```python
from build123d import *

# Parameters (mm, degrees)
SKETCH050_W      = 37
SKETCH050_H      = 132
PAD_DEPTH        = 6
PAD_DEPTH_BACK   = 4
SKETCH051_W      = 37
SKETCH051_H      = 119
POCKET006_DEPTH  = 4
HOLE_D           = 2.4
HOLE_DEPTH       = 25
HOLE_CBORE_D     = 3.5
HOLE_CBORE_DEPTH = 2.1
BINDER020_W      = 119
BINDER020_H      = 64
PAD012_DEPTH     = 6
SKETCH_R         = 1.75
POCKET_DEPTH     = 9
POCKET001_DEPTH  = 5
POCKET002_DEPTH  = 5
SKETCH046_R      = 1.75
POCKET003_DEPTH  = 4
POCKET004_DEPTH  = 5
SKETCH048_R      = 1.75
POCKET005_DEPTH  = 4


with BuildPart() as obj1:
    # Sketch050 (on Face1 of Binder) → Pad (new body, two sides)
    with BuildSketch(Plane.XY) as pad_sk:
        with Locations((-13.5, 0)):
            Rectangle(SKETCH050_W, SKETCH050_H)
    extrude(amount=PAD_DEPTH)
    extrude(pad_sk.sketch, amount=-PAD_DEPTH_BACK)

    # Sketch051 (on Face5 of Pad) → Pocket006 (cut)
    with BuildSketch(Plane(origin=(0, 0, -4), x_dir=(1, 0, 0), z_dir=(0, 0, -1))):
        with Locations((-13.5, 0)):
            Rectangle(SKETCH051_W, SKETCH051_H)
    extrude(amount=-POCKET006_DEPTH, mode=Mode.SUBTRACT)

    # Hole
    with Locations(Plane.XY.offset(6)):
        with Locations((-28.75, 62.75), (1.75, 62.75), (-28.75, -62.75), (1.75, -62.75)):
            CounterBoreHole(HOLE_D / 2, HOLE_CBORE_D / 2, HOLE_CBORE_DEPTH, depth=HOLE_DEPTH)


with BuildPart() as fusion:
    # Binder020 → Pad012 (new body)
    with BuildSketch(Plane(origin=(0, 0, 0), x_dir=(0, 1, 0), z_dir=(0, 0, 1))):
        Rectangle(BINDER020_W, BINDER020_H)
    extrude(amount=PAD012_DEPTH)

    # Sketch (on Face2 of Pad012) → Pocket (cut)
    with BuildSketch(Plane.YZ.offset(32)):
        with Locations((-34.5, 3)):
            Circle(SKETCH_R)
        with Locations((34.5, 3)):
            Circle(SKETCH_R)
    extrude(amount=-POCKET_DEPTH, mode=Mode.SUBTRACT)

    # Sketch044 (on Face3 of Pocket) → Pocket001 (cut)
    with BuildSketch(Plane.YZ.offset(32)):
        Polygon((-40.5, 0), (-38.316179, 6), (-30.683821, 6), (-28.5, 0), align=None)
        Polygon((30.683821, 6), (38.316179, 6), (40.5, 0), (28.5, 0), align=None)
    extrude(amount=-POCKET001_DEPTH, mode=Mode.SUBTRACT)

    # Sketch045 (on Face1 of Pocket001) → Pocket002 (cut)
    with BuildSketch(Plane.XZ.offset(59.5)):
        Polygon((10, 0), (12.183821, 6), (19.816179, 6), (22, 0), align=None)
    extrude(amount=-POCKET002_DEPTH, mode=Mode.SUBTRACT)

    # Sketch046 (on Face18 of Pocket002) → Pocket003 (cut)
    with BuildSketch(Plane.XZ.offset(54.5)):
        with Locations((16, 3)):
            Circle(SKETCH046_R)
    extrude(amount=-POCKET003_DEPTH, mode=Mode.SUBTRACT)

    # Sketch047 (on Face6 of Pocket003) → Pocket004 (cut)
    with BuildSketch(Plane(origin=(0, 59.5, 0), x_dir=(-1, 0, 0), z_dir=(0, 1, 0))):
        Polygon((-22, 0), (-19.816179, 6), (-12.183821, 6), (-10, 0), align=None)
    extrude(amount=-POCKET004_DEPTH, mode=Mode.SUBTRACT)

    # Sketch048 (on Face20 of Pocket004) → Pocket005 (cut)
    with BuildSketch(Plane(origin=(0, 54.5, 0), x_dir=(-1, 0, 0), z_dir=(0, 1, 0))):
        with Locations((-16, 3)):
            Circle(SKETCH048_R)
    extrude(amount=-POCKET005_DEPTH, mode=Mode.SUBTRACT)

    # Fusion: union obj1
    add(obj1.part)


solid = fusion.part
```
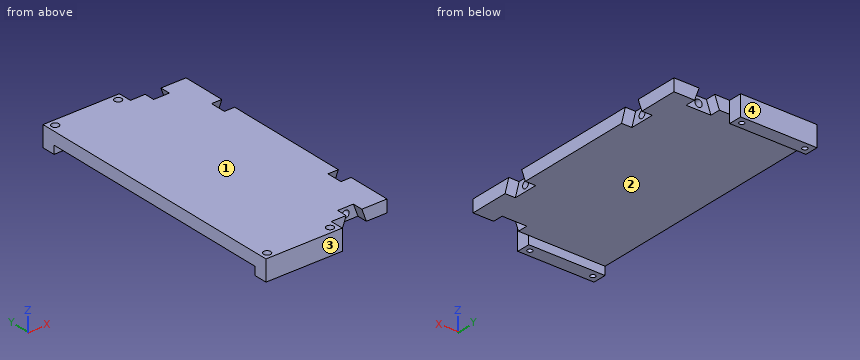
Part model, mm, in its own coordinate system. Face numbers are marked on the shaded views. Round coordinates to 2 decimals unless told otherwise and drop trailing zeros. Loops run counter-clockwise (first coordinate to the right, second up) from the corner with the lowest first, then second, coordinate; pieces in that order, holes last. Notation, with made-up numbers: (19, -18) -> (47, -18) arc R32 ccw to (47, 9) -> close; hole circle Ø2 at (11.25, 17). An arc over 180 degrees is marked (long way). Use one line per item in the form item = value. Start each with the question number.
Item 1: Band-saw the part on C-C (x = -28.75). List the corners of the cut face in (y, z), plus the area to 3 significant figures.
Item 2: Two-plate mould, pull along Y, no slides. Class the marked faces 1, 2, 3 and 4: released by +Y, released by -Y, zero draft, split by the parting line, or undercut.
Item 3: Band-saw the part on A-A (z = -1.5). List the corners of the cut face in (x, y).
Item 4: Drill centre lines: line 1 along Y through (x, z) = (1.75, 0.75); line 2 along Y through (x, z) = (1.75, 4.8); line 3 along Y through (x, z) = (-22.5, -3). Where is each one in solid material? Low to high.
Item 5: Band-saw the part on B-B (x = 16). List the corners of the cut face in (y, z), plus the area to 3 significant figures.
Item 6: Drop flat-ended pins along their axis: pin 1 Ø1.5 at (x, z) = (7, -1) entering from -Y; pin 2 Ø1.8 at (x, z) = (16, 3) entering from +Y; pin 3 Ø2 at (x, y) = (0.5, 16.5) entering from -Z; pin 4 Ø5 at (x, z) = (10, 2.5) entering from -Y. Give the stop position or say it passes through.
Item 7: Band-saw the part on D-D (y = -34.5). List the corners of the cut face in (x, z), plus the area to 3 significant figures.
Data:
q1.outline = (-66, -4) -> (-63.95, -4) -> (-63.95, 3.9) -> (-64.5, 3.9) -> (-64.5, 6) -> (-66, 6) -> close; (-61.55, -4) -> (-59.5, -4) -> (-59.5, 0) -> (59.5, 0) -> (59.5, -4) -> (61.55, -4) -> (61.55, 3.9) -> (61, 3.9) -> (61, 6) -> (-61, 6) -> (-61, 3.9) -> (-61.55, 3.9) -> close; (63.95, -4) -> (66, -4) -> (66, 6) -> (64.5, 6) -> (64.5, 3.9) -> (63.95, 3.9) -> close
q1.area = 791 mm^2
q2.face_1 = zero draft
q2.face_2 = undercut
q2.face_3 = released by -Y
q2.face_4 = released by +Y
q3.outline = (-32, -66) -> (5, -66) -> (5, -59.5) -> (-32, -59.5) -> close; (-32, 59.5) -> (5, 59.5) -> (5, 66) -> (-32, 66) -> close; hole circle Ø2.4 at (-28.75, -62.75); hole circle Ø2.4 at (-28.75, 62.75); hole circle Ø2.4 at (1.75, -62.75); hole circle Ø2.4 at (1.75, 62.75)
q4.line_1 = -66 to -63.95, -61.55 to 61.55, 63.95 to 66
q4.line_2 = -66 to -64.5, -61 to 61, 64.5 to 66
q4.line_3 = -66 to -59.5, 59.5 to 66
q5.outline = (-54.5, 0) -> (54.5, 0) -> (54.5, 1.25) -> (50.5, 1.25) -> (50.5, 4.75) -> (54.5, 4.75) -> (54.5, 6) -> (-54.5, 6) -> (-54.5, 4.75) -> (-50.5, 4.75) -> (-50.5, 1.25) -> (-54.5, 1.25) -> close
q5.area = 626 mm^2
q6.pin_1 = through
q6.pin_2 = 50.5
q6.pin_3 = 0
q6.pin_4 = -59.5
q7.outline = (-32, 0) -> (27, 0) -> (27, 1.25) -> (23, 1.25) -> (23, 4.75) -> (27, 4.75) -> (27, 6) -> (-32, 6) -> close
q7.area = 340 mm^2
